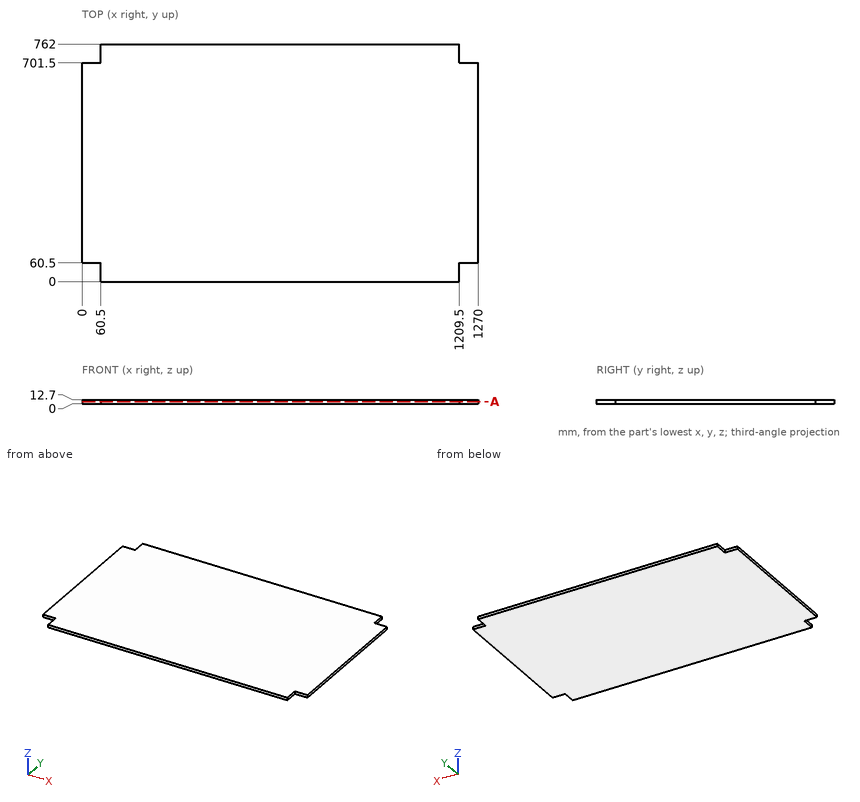
Geometry check sheet. Reference: drawing and pictorial views, mm from the part's lowest x, y, z. Give positions to 0.01 mm unless a question says otherwise; leave off trailing zeros. Write each loop counter-clockwise with the first axis right and the second up, starting at its lowest first coordinate (ties: lowest second). Pieces come first, ordered by that corner, then holes. Notation, with made-up numbers: (45.25, -13) -> (85.25, -13) arc R28 cw to (85.25, 23) -> close; hole circle Ø4 at (48.25, 63). An arc over 180 degrees is marked (long way). One line per item, written item: value. Start each with the question number.
Item 1: Material ranges on probe 1 along X at (y, z) = (46, 2.25), recorded low to high. Write a range as from..to.
Item 2: Section check A-A on z = 6.5. Record the cut outline in (x, y).
Item 3: Gauge pin test, flat ends, axial feed: pin 1 (4 mm diameter, centred on y = 744.5, z = 4, fed in from +X); pin 2 (6.5 mm diameter, centred on y = 28, z = 7, fed in from -X); pin 3 (12 mm diameter, centred on x = 864.5, y = 102, fed in from -Z). Record the tip position at first contact, or that the pin passes through.
Results list:
1. probe 1: 60.5..1209.5
2. outline: (0, 60.5) -> (60.5, 60.5) -> (60.5, 0) -> (1209.5, 0) -> (1209.5, 60.5) -> (1270, 60.5) -> (1270, 701.5) -> (1209.5, 701.5) -> (1209.5, 762) -> (60.5, 762) -> (60.5, 701.5) -> (0, 701.5) -> close
3. pin 1: x = 1209.5
3. pin 2: x = 60.5
3. pin 3: z = 0
